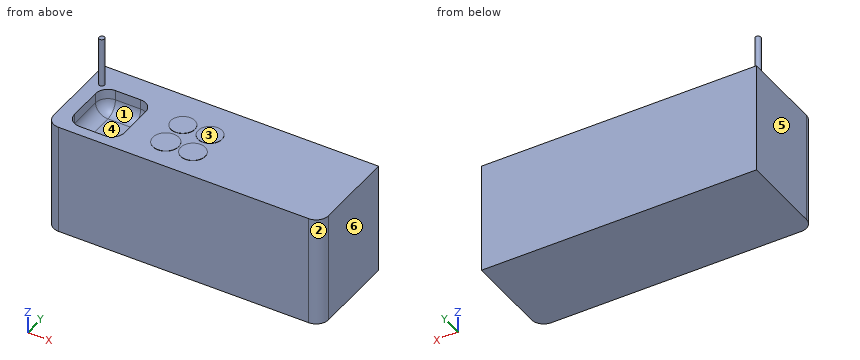
```python
from build123d import *

# Parameters (mm, degrees)
F1_DEPTH = 45
F2_R     = 4.8450580426
F2_R_2   = 4.845014418
F2_R_3   = 5.2193072221
F2_R_4   = 4.9662241181
F3_DEPTH = 0.1
F4_DEPTH = 9
F5_R     = 5
F2_R_5   = 1.0935604598
F6_DEPTH = 20


with BuildPart() as f1:
    # F0 (on Top) → F1 (new body)
    with BuildSketch(Plane.XY):
        with BuildLine():
            Line((60.0371286273, 18.452970311), (-50.9405955672, 18.452970311))
            Line((-50.9405955672, 18.452970311), (-50.9405955672, -14.7524763644))
            ThreePointArc((-50.9405955672, -14.7524763644), (-49.4761294732, -18.2880102703), (-45.9405955672, -19.7524763644))
            Line((-45.9405955672, -19.7524763644), (55.0371286273, -19.7524763644))
            ThreePointArc((55.0371286273, -19.7524763644), (58.5726625332, -18.2880102703), (60.0371286273, -14.7524763644))
            Line((60.0371286273, -14.7524763644), (60.0371286273, 18.452970311))
        make_face()
    extrude(amount=F1_DEPTH)

    # F2 (on face) → F3 (join)
    with BuildSketch(Plane.XY.offset(45)):
        with Locations((1.0965270922, 3.5560266115)):
            Circle(F2_R)
        with Locations((-9.8790517077, 3.5560266115)):
            Circle(F2_R_2)
        with Locations((-9.8790517077, -7.8143570572)):
            Circle(F2_R_3)
        with Locations((1.0965270922, -7.8143570572)):
            Circle(F2_R_4)
    extrude(amount=F3_DEPTH)

    # F2 (on face) → F4 (cut)
    with BuildSketch(Plane.XY.offset(45)):
        with BuildLine():
            Line((-29.8118992895, 8.4029044956), (-40.030772686, 8.4029044956))
            ThreePointArc((-40.030772686, 8.4029044956), (-43.5663065919, 6.9384384015), (-45.030772686, 3.4029044956))
            Line((-45.030772686, 3.4029044956), (-45.030772686, -10.5901564285))
            ThreePointArc((-45.030772686, -10.5901564285), (-43.5663065919, -14.1256903344), (-40.030772686, -15.5901564285))
            Line((-40.030772686, -15.5901564285), (-29.8118992895, -15.5901564285))
            ThreePointArc((-29.8118992895, -15.5901564285), (-26.2763653836, -14.1256903344), (-24.8118992895, -10.5901564285))
            Line((-24.8118992895, -10.5901564285), (-24.8118992895, 3.4029044956))
            ThreePointArc((-24.8118992895, 3.4029044956), (-26.2763653836, 6.9384384015), (-29.8118992895, 8.4029044956))
        make_face()
    extrude(amount=-F4_DEPTH, mode=Mode.SUBTRACT)

    # F5
    f5_edges = [f1.edges().sort_by_distance(p)[0] for p in [
        (-43.566307, 6.938438, 36),
        (-34.921336, 8.402904, 36),
    ]]
    fillet(f5_edges, radius=F5_R)

    # F2 (on face) → F6 (join)
    with BuildSketch(Plane.XY.offset(45)):
        with Locations((-45.9486916661, 9.11985524)):
            Circle(F2_R_5)
    extrude(amount=F6_DEPTH)


solid = f1.part
```
The model under review builds one solid part; all positions refer to its coordinate system, in mm. Face numbers are marked on the shaded views. A direction names the side the tool comes from. Give positions to 0.01 mm unless a question says otherwise; leave off trailing zeros. Order: outer loops, then holes, each group sorted by start corner. A loop starts at its lowest first (then second) coordinate and runs counter-clockwise, first axis right, second up. Notation, with made-up numbers: (26.5, 7) - (78.5, 7) arc R28 ccw to (78.5, 27) - close; hole circle Ø10 at (43.25, 86). An arc over 180 degrees is marked (long way). Use CSV: the item, a comma, the result in double quotes. Start each with the question number.
Q1. We need section D-D, the plane x = 4. Write out the cut boundary in (y, z).
Q2. To check wall thickness, follow line 1 along X through (y, z) = (-1, 44); line 2 along Z through (x, y) = (42.5, -6); line 3 along Z through (x, y) = (-37, 2). State the ranges of each line that lie inside material, in increasing order. Write a range as [from, to].
Q3. The part is to be moulded in two halves that separate along X. For the marked faces 3, 4, 5 and 6, say which applies: +X half, -X half, draft (parallel to the pull), parting line (faces both ways), or undercut.
Q4. We need section B-B, the plane x = -43. Write out the cut boundary in (y, z), and give its area (3 significant figures).
Q5. We need section A-A, the plane z = 43. Write out the cut boundary in (x, y).
Q6. Clearance check with flat-ended pins moving along their axes: pin 1 Ø5 at (x, y) = (-10.5, 4) entering from +Z; pin 2 Ø8 at (x, y) = (-36, -6) entering from +Z; pin 3 Ø6 at (x, z) = (46.5, 47.5) entering from +Y; pin 4 Ø19 at (x, y) = (21.5, -3) entering from +Z. State where each tip first meets the part, or that it passes through.
Q7. We need section C-C, the plane z = 52.5. Write out the cut boundary in (x, y), and give its area (3 significant figures).
Q8. Tool access review of the marked faces 1 and 2: name each direction out of +Z, -Z, +X, -X, +Y, -Y from which nothing blocks a thin tool from reaching the whole face with its end or side.
Outcome:
1,outline,"(-19.75, 0) - (18.45, 0) - (18.45, 45) - (7.43, 45) - (7.43, 45.1) - (-0.32, 45.1) - (-0.32, 45) - (-3.79, 45) - (-3.79, 45.1) - (-11.84, 45.1) - (-11.84, 45) - (-19.75, 45) - close"
2,line 1,"x = [-50.94, -45.03], [-24.81, 60.04]"
2,line 2,"z = [0, 45]"
2,line 3,"z = [0, 36]"
3,face 3,"draft"
3,face 4,"undercut"
3,face 5,"-X half"
3,face 6,"+X half"
4,outline,"(-19.75, 0) - (18.45, 0) - (18.45, 45) - (7.43, 45) - (7.43, 41) arc R4.02 cw to (3.4, 36.98) - (-10.59, 36.98) arc R4.02 cw to (-14.61, 41) - (-14.61, 45) - (-19.75, 45) - close"
4,area,"1,550 mm^2"
5,outline,"(-50.94, -14.75) arc R5 ccw to (-45.94, -19.75) - (55.04, -19.75) arc R5 ccw to (60.04, -14.75) - (60.04, 18.45) - (-50.94, 18.45) - close; hole (-45.03, -10.59) arc R5 ccw to (-40.03, -15.59) - (-29.81, -15.59) arc R5 ccw to (-24.81, -10.59) - (-24.81, 3.4) arc R5 ccw to (-29.81, 8.4) - (-40.03, 8.4) arc R5 ccw to (-45.03, 3.4) - close"
6,pin 1,"stops at z = 45.1"
6,pin 2,"stops at z = 36"
6,pin 3,"stops at y = 18.45"
6,pin 4,"stops at z = 45"
7,outline,"circle Ø2.19 at (-45.95, 9.12)"
7,area,"3.76 mm^2"
8,face 1,"+Z"
8,face 2,"+Z, -Z, +X, -Y"
